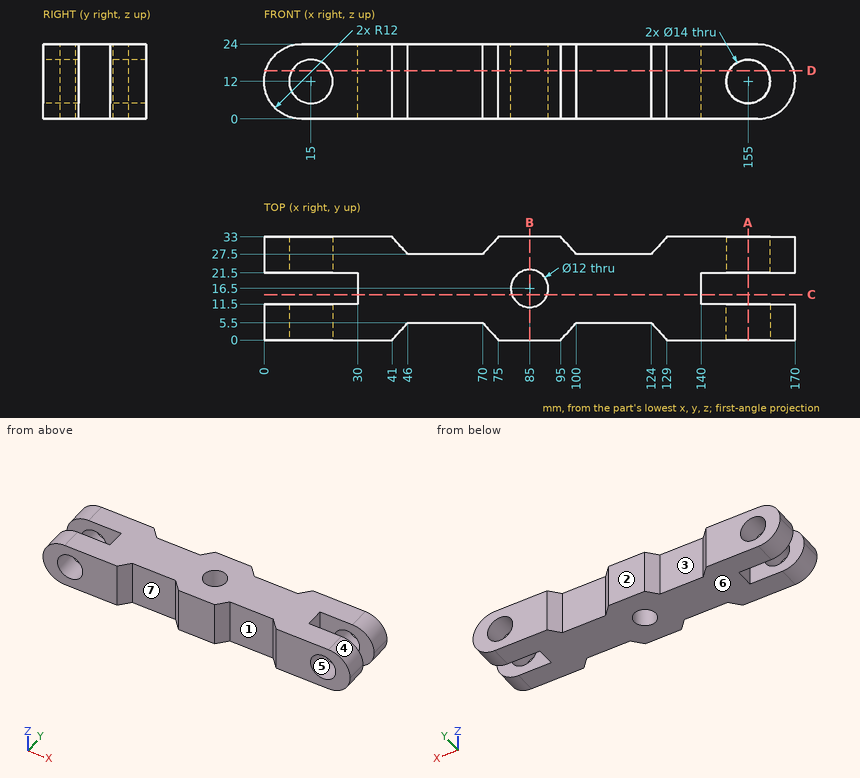
Drawing for the job (mm, zero at the part's lowest x, y, z). A direction names the side the tool comes from. Round coordinates to 2 decimals unless told otherwise and drop trailing zeros. Order: outer loops, then holes, each group sorted by start corner. A loop starts at its lowest first (then second) coordinate and runs counter-clockwise, first axis right, second up. Notation, with made-up numbers: (71, 17) -> (86, 17) arc R21 ccw to (86, 22) -> close; hole circle Ø3 at (76, 70.5). An arc over 180 degrees is marked (long way). Put each result on its own line as item: value.
Q1. Wall check: line 1 (X direction, y = 11, z = 15.25); line 2 (Y direction, x = 85, z = 13.75); line 3 (Z direction, x = 15, y = 27). Give the ranges that are in metal, low to high. Write a range as [from, to].
From the geometry:
line 1: x = [0.45, 8.8], [21.2, 82.6], [87.4, 148.8], [161.2, 169.55]
line 2: y = [0, 10.5], [22.5, 33]
line 3: z = [0, 5], [19, 24]
Q2. Tool access for the marked faces 1, 2 and 3: list every direction of +Z, -Z, +X, -X, +Y, -Y with a clear straight run to the whole face (end or side of a thin tool).
From the geometry:
face 1: +Z, -Z, -Y
face 2: +Z, -Z, +X, -X, +Y
face 3: +Z, -Z, +Y
Q3. Band-saw the part on B-B (x = 85). Give the cut face in (y, z).
From the geometry:
outline: (0, 0) -> (10.5, 0) -> (10.5, 24) -> (0, 24) -> close; (22.5, 0) -> (33, 0) -> (33, 24) -> (22.5, 24) -> close
Q4. Pin check, flat tips, straight feed: pin 1 Ø1 at (y, z) = (7, 10.5) entering from -X; pin 2 Ø2 at (y, z) = (4.5, 17) entering from +X; pin 3 Ø7 at (x, z) = (8.5, 16) entering from -Y; pin 4 Ø5 at (y, z) = (16.5, 10) entering from +X. Stop position of each tip, or through.
From the geometry:
pin 1: stops at x = 0.04
pin 2: stops at x = 169.31
pin 3: stops at y = 0
pin 4: stops at x = 140
Q5. Band-saw the part on A-A (x = 155). Give the cut face in (y, z), and give its area (3 significant figures).
From the geometry:
outline: (0, 0) -> (11.5, 0) -> (11.5, 5) -> (0, 5) -> close; (0, 19) -> (11.5, 19) -> (11.5, 24) -> (0, 24) -> close; (21.5, 0) -> (33, 0) -> (33, 5) -> (21.5, 5) -> close; (21.5, 19) -> (33, 19) -> (33, 24) -> (21.5, 24) -> close
area: 230 mm2
Q6. Band-saw the part on D-D (z = 15.5). State how many separate pieces and enclosed holes the cut face has, and give its area (3 significant figures).
From the geometry:
separate pieces: 5
enclosed holes: 1
area: 3,680 mm2
Q7. Band-saw the part on C-C (y = 14.5). Give the cut face in (x, z).
From the geometry:
outline: (30, 0) -> (79.34, 0) -> (79.34, 24) -> (30, 24) -> close; (90.66, 0) -> (140, 0) -> (140, 24) -> (90.66, 24) -> close
Q8. Pull direction X, two halves, no side cores. Call the marked faces 4, 5, 6 and 7: pulls with the +X half, pulls with the -X half, needs draft (parallel to the pull), parting line crosses it, or undercut.
From the geometry:
face 4: pulls with the +X half
face 5: undercut
face 6: needs draft
face 7: undercut
